from build123d import *

# Parameters (mm, degrees)
F0_R         = 15
F1_DEPTH     = 20
F2_R         = 5
F3_T1_DEPTH  = 24.0817816001
F3_T6_DEPTH  = 5
F3_T12_DEPTH = 5
F3_T18_DEPTH = 5
F3_T24_DEPTH = 5
F3_T30_DEPTH = 5
F4_DEPTH     = 34.1


# Not quite as in the source:
# - a fillet or chamfer that OpenCascade refuses, or shapes differently, is made with other operations: its cross-section is extruded or revolved along the edge and cut away or added


with BuildPart() as f1:
    # F0 (on Front) → F1 (new body)
    with BuildSketch(Plane.XZ):
        Polygon((-20, -27.5276384094), (20, -27.5276384094), (32.360679775, 10.5146222424), (0, 34.0260323341), (-32.360679775, 10.5146222424), align=None)
        Circle(F0_R, mode=Mode.SUBTRACT)
    extrude(amount=F1_DEPTH)

    # F2
    f2_edges = [f1.edges().sort_by_distance(p)[0] for p in [
        (-26.18034, -20, -8.506508),
        (0, -20, -27.527638),
        (26.18034, -20, -8.506508),
        (16.18034, -20, 22.270327),
        (-16.18034, -20, 22.270327),
    ]]
    fillet(f2_edges, radius=F2_R)

    # F3: fillet of radius 5 on 5 edges, made by hand

    # F3_s2 → F3_t1 (cut)
    with BuildSketch(Plane.XZ.offset(-9.0817816001)):
        with BuildLine():
            ThreePointArc((16.36728736, -27.5276384094), (19.3062136214, -26.5727233813), (21.1225699414, -24.0727233813))
            Line((21.1225699414, -24.0727233813), (20, -27.5276384094))
            Line((20, -27.5276384094), (16.36728736, -27.5276384094))
        make_face()
        with BuildLine():
            ThreePointArc((29.4217535135, 12.649877158), (31.2381098335, 10.149877158), (31.2381098335, 7.0597072143))
            Line((31.2381098335, 7.0597072143), (32.360679775, 10.5146222424))
            Line((32.360679775, 10.5146222424), (29.4217535135, 12.649877158))
        make_face()
        with BuildLine():
            ThreePointArc((-2.9389262615, 31.8907774185), (0, 32.8456924466), (2.9389262615, 31.8907774185))
            Line((2.9389262615, 31.8907774185), (0, 34.0260323341))
            Line((0, 34.0260323341), (-2.9389262615, 31.8907774185))
        make_face()
        with BuildLine():
            ThreePointArc((-31.2381098335, 7.0597072143), (-31.2381098335, 10.149877158), (-29.4217535135, 12.649877158))
            Line((-29.4217535135, 12.649877158), (-32.360679775, 10.5146222424))
            Line((-32.360679775, 10.5146222424), (-31.2381098335, 7.0597072143))
        make_face()
        with BuildLine():
            ThreePointArc((-21.1225699414, -24.0727233813), (-19.3062136214, -26.5727233813), (-16.36728736, -27.5276384094))
            Line((-16.36728736, -27.5276384094), (-20, -27.5276384094))
            Line((-20, -27.5276384094), (-21.1225699414, -24.0727233813))
        make_face()
    extrude(amount=F3_T1_DEPTH, mode=Mode.SUBTRACT)


with BuildPart() as f3_tool4:
    # F3_s5 → F3_t6 (new body)
    with BuildSketch(Plane.XZ.offset(15)):
        Polygon((-16.36728736, -22.5276384094), (-21.1225699414, -24.0727233813), (-20, -27.5276384094), (-16.36728736, -27.5276384094), align=None)
    extrude(amount=F3_T6_DEPTH)

    # F3_s7 → F3_t8 (revolve, cut)
    with BuildSketch(Plane(origin=(-16.36728736, -15, -22.5276384094), x_dir=(0.5877852523, 0, 0.8090169944), z_dir=(0.8090169944, 0, -0.5877852523))):
        with BuildLine():
            ThreePointArc((0, -5), (5, 0), (0, 5))
            Line((0, 5), (0, -5))
        make_face()
    revolve(axis=Axis((-16.36728736, -15, -22.5276384094), (0, -1, 0)), mode=Mode.SUBTRACT)


with BuildPart() as f1_1:
    add(f1.part)

    # F3_t3: cut F3_tool4
    add(f3_tool4.part, mode=Mode.SUBTRACT)


with BuildPart() as f3_tool10:
    # F3_s11 → F3_t12 (new body)
    with BuildSketch(Plane.XZ.offset(15)):
        Polygon((-26.4828272521, 8.6047921861), (-31.2381098335, 7.0597072143), (-32.360679775, 10.5146222424), (-29.4217535135, 12.649877158), align=None)
    extrude(amount=F3_T12_DEPTH)

    # F3_s13 → F3_t14 (revolve, cut)
    with BuildSketch(Plane(origin=(-26.4828272521, -15, 8.6047921861), x_dir=(0.9510565163, 0, -0.3090169944), z_dir=(-0.3090169944, 0, -0.9510565163))):
        with BuildLine():
            ThreePointArc((0, -5), (5, 0), (0, 5))
            Line((0, 5), (0, -5))
        make_face()
    revolve(axis=Axis((-26.4828272521, -15, 8.6047921861), (0, -1, 0)), mode=Mode.SUBTRACT)


with BuildPart() as f1_2:
    add(f1_1.part)

    # F3_t9: cut F3_tool10
    add(f3_tool10.part, mode=Mode.SUBTRACT)


with BuildPart() as f3_tool16:
    # F3_s17 → F3_t18 (new body)
    with BuildSketch(Plane.XZ.offset(15)):
        Polygon((0, 27.8456924466), (-2.9389262615, 31.8907774185), (0, 34.0260323341), (2.9389262615, 31.8907774185), align=None)
    extrude(amount=F3_T18_DEPTH)

    # F3_s19 → F3_t20 (revolve, cut)
    with BuildSketch(Plane(origin=(0, -15, 27.8456924466), x_dir=(0, 0, -1), z_dir=(-1, 0, 0))):
        with BuildLine():
            ThreePointArc((0, -5), (5, 0), (0, 5))
            Line((0, 5), (0, -5))
        make_face()
    revolve(axis=Axis((0, -15, 27.8456924466), (0, -1, 0)), mode=Mode.SUBTRACT)


with BuildPart() as f1_3:
    add(f1_2.part)

    # F3_t15: cut F3_tool16
    add(f3_tool16.part, mode=Mode.SUBTRACT)


with BuildPart() as f3_tool22:
    # F3_s23 → F3_t24 (new body)
    with BuildSketch(Plane.XZ.offset(15)):
        Polygon((26.4828272521, 8.6047921861), (29.4217535135, 12.649877158), (32.360679775, 10.5146222424), (31.2381098335, 7.0597072143), align=None)
    extrude(amount=F3_T24_DEPTH)

    # F3_s25 → F3_t26 (revolve, cut)
    with BuildSketch(Plane(origin=(26.4828272521, -15, 8.6047921861), x_dir=(-0.9510565163, 0, -0.3090169944), z_dir=(-0.3090169944, 0, 0.9510565163))):
        with BuildLine():
            ThreePointArc((0, -5), (5, 0), (0, 5))
            Line((0, 5), (0, -5))
        make_face()
    revolve(axis=Axis((26.4828272521, -15, 8.6047921861), (0, -1, 0)), mode=Mode.SUBTRACT)


with BuildPart() as f1_4:
    add(f1_3.part)

    # F3_t21: cut F3_tool22
    add(f3_tool22.part, mode=Mode.SUBTRACT)


with BuildPart() as f3_tool28:
    # F3_s29 → F3_t30 (new body)
    with BuildSketch(Plane.XZ.offset(15)):
        Polygon((16.36728736, -22.5276384094), (16.36728736, -27.5276384094), (20, -27.5276384094), (21.1225699414, -24.0727233813), align=None)
    extrude(amount=F3_T30_DEPTH)

    # F3_s31 → F3_t32 (revolve, cut)
    with BuildSketch(Plane(origin=(16.36728736, -15, -22.5276384094), x_dir=(-0.5877852523, 0, 0.8090169944), z_dir=(0.8090169944, 0, 0.5877852523))):
        with BuildLine():
            ThreePointArc((0, -5), (5, 0), (0, 5))
            Line((0, 5), (0, -5))
        make_face()
    revolve(axis=Axis((16.36728736, -15, -22.5276384094), (0, -1, 0)), mode=Mode.SUBTRACT)


with BuildPart() as f1_5:
    add(f1_4.part)

    # F3_t27: cut F3_tool28
    add(f3_tool28.part, mode=Mode.SUBTRACT)

    # F0 (on Front) → F4 (join)
    with BuildSketch(Plane.XZ):
        Circle(F0_R)
    extrude(amount=F4_DEPTH)

    # F5: chamfer of 15 on 1 edges, made by hand


with BuildPart() as f5_tool2:
    # F5_s3 → F5_t4 (revolve)
    with BuildSketch(Plane.XY):
        Polygon((15, -19.1), (0, -34.1), (15, -34.1), align=None)
    revolve(axis=Axis((0, -34.1, 0), (0, -1, 0)))

    split(bisect_by=Plane.XZ.offset(20), keep=Keep.TOP)


with BuildPart() as f1_6:
    add(f1_5.part)

    # F5_t1: cut F5_tool2
    add(f5_tool2.part, mode=Mode.SUBTRACT)


solid = f1_6.part
Model file for the job. Use its own axes, mm. A direction names the side the tool comes from. Coordinates: 2 decimals unless noted, no trailing zeros. Write each loop counter-clockwise with the first axis right and the second up, starting at its lowest first coordinate (ties: lowest second). Pieces come first, ordered by that corner, then holes. Notation, with made-up numbers: (-13, 16.5) - (-4, 16.5) arc R30 ccw to (-4, 41.5) - close; hole circle Ø10 at (80, -28.5). An arc over 180 degrees is marked (long way). Write each question's results on one line, items separated by ' | '. Start each with the question number.
1) Cut at B-B (y = -28). Write the cut outline in (x, z).
2) Probe line 1 along Y through (x, z) = (-4, -16.5); line 2 along X through (y, z) = (-19, 27.5); line 3 along Y through (x, z) = (28, 9). List the from-to ranges inside material, lowest first. Write a range as from..to.
3) 3-axis set-ups, long thin cutter, end or side, ignore diameter. For faces 1 (the face through (24.895, -18.496, -7.848)), 2 (the face through (11.4, -20, 8.6)): which of +Z, -Z, +X, -X, +Y, -Y reach the whole face in a straight line?
4) Flat gauge pins, fed straight in: P1, Ø2, axis at x = -16, y = -22, coming from the +Z side; P2, Ø1.5, axis at x = -3.5, y = -17, coming from the +Z side; P3, Ø10, axis at y = -9, z = 18.5, coming from the +X side; P4, Ø4, axis at y = -11, z = 11, coming from the +X side. Where does each tip first touch, or does it go through?
5) Cut at A-A (y = -3.5). Write the cut outline in (x, z), then the cut area to 3 significant figures.
Returned:
1) outline: circle Ø12.2 at (0, 0)
2) line 1: -20..0 | line 2: -5.58..5.58 | line 3: -19.75..0
3) face 1: -Z, +X, -Y | face 2: -Y
4) P1: through | P2: z = 31.62 | P3: x = 28.25 | P4: x = 31.47
5) outline: (-31.24, 7.06) - (-21.12, -24.07) arc R5 ccw to (-16.37, -27.53) - (16.37, -27.53) arc R5 ccw to (21.12, -24.07) - (31.24, 7.06) arc R5 ccw to (29.42, 12.65) - (2.94, 31.89) arc R5 ccw to (-2.94, 31.89) - (-29.42, 12.65) arc R5 ccw to start | area: 2,740 mm^2
